Check sheet for the drawn part. Datum: minimum x, y, z corner. Units: mm. A direction names the side the tool comes from. Give positions to 0.01 mm unless a question says otherwise; leave off trailing zeros. Order: outer loops, then holes, each group sorted by start corner. A loop starts at its lowest first (then second) coordinate and runs counter-clockwise, first axis right, second up.
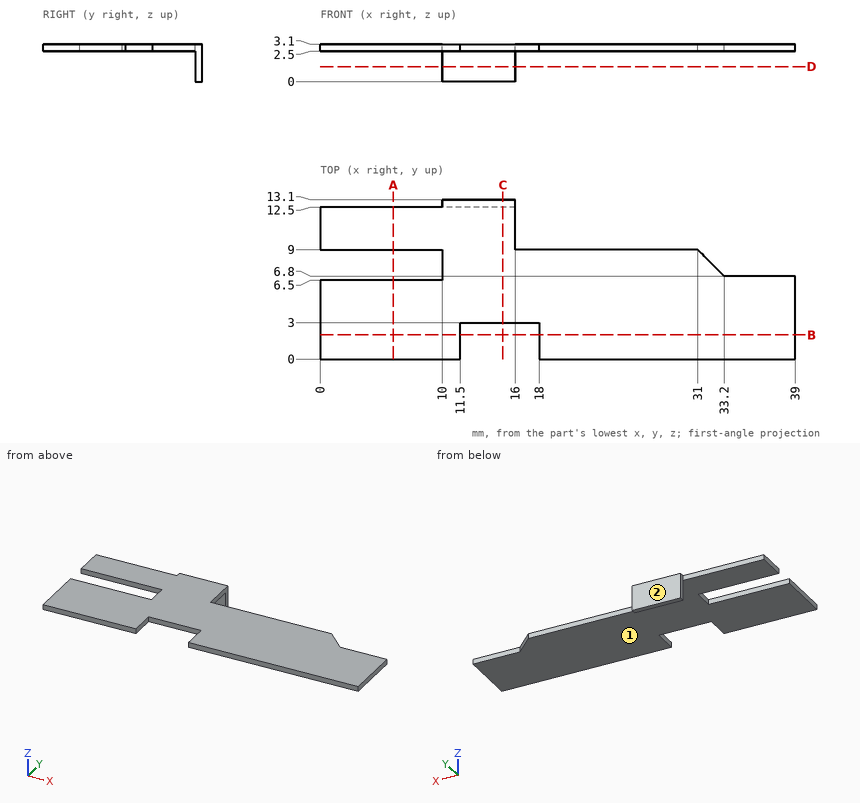
Item 1: Scan lines: L1, parallel to Y at x = 3, z = 2.7; L2, parallel to Y at x = 14.5, z = 1.15; L3, parallel to X at y = 11, z = 3.05. Record each from-to range of solid material in increasing order.
Reported:
L1: y = 0 to 6.5, 9 to 12.5
L2: y = 12.5 to 13.1
L3: x = 0 to 16
Item 2: Gauge pin test, flat ends, axial feed: pin 1 (0.7 mm diameter, centred on x = 3.5, z = 3, fed in from +Y); pin 2 (6 mm diameter, centred on x = 13, y = 3.5, fed in from -Z); pin 3 (0.5 mm diameter, centred on x = 15.5, z = 3, fed in from -Y). Record the tip position at first contact, or that the pin passes through.
Reported:
pin 1: stops at y = 12.5
pin 2: stops at z = 2.5
pin 3: stops at y = 3
Item 3: Set-up check for the marked faces 1 and 2: record each of +Z, -Z, +X, -X, +Y, -Y from which the full face is reachable in a straight line by a thin tool's end or side.
Reported:
face 1: -Z, +X, -X, -Y
face 2: +Z, -Z, +X, -X, +Y
Item 4: Sectioned sample at A-A (x = 6). Enter the section's corners in (y, z), and give its area (3 significant figures).
Reported:
outline: (0, 2.5) - (6.5, 2.5) - (6.5, 3.1) - (0, 3.1) - close; (9, 2.5) - (12.5, 2.5) - (12.5, 3.1) - (9, 3.1) - close
area: 6.00 mm2
Item 5: Sectioned sample at C-C (x = 15). Enter the section's corners in (y, z), and give its area (3 significant figures).
Reported:
outline: (3, 2.5) - (12.5, 2.5) - (12.5, 0) - (13.1, 0) - (13.1, 3.1) - (3, 3.1) - close
area: 7.56 mm2
Item 6: Sectioned sample at B-B (y = 2). Enter the section's corners in (x, z).
Reported:
outline: (0, 2.5) - (11.5, 2.5) - (11.5, 3.1) - (0, 3.1) - close; (18, 2.5) - (39, 2.5) - (39, 3.1) - (18, 3.1) - close
Item 7: Sectioned sample at D-D (z = 1.25). Enter the section's corners in (x, y), and give its area (3 significant figures).
Reported:
outline: (10, 12.5) - (16, 12.5) - (16, 13.1) - (10, 13.1) - close
area: 3.60 mm2
